Input: part model. Units: mm. Frame: model coordinates. Face numbers are marked on the shaded views. A direction names the side the tool comes from. Coordinates: 2 decimals unless noted, no trailing zeros. Loops run counter-clockwise (first coordinate to the right, second up) from the corner with the lowest first, then second, coordinate; pieces in that order, holes last.
Item 1: Reachability of the marked faces 3 and 4 from +Z, -Z, +X, -X, +Y, -Y: full face, straight path, thin tool, end or side. Return the list, or none.
Item 2: Section A-A on y = 32. Return loops of the section in (x, z).
Item 3: Pull-direction query (Z, two-part tool) for the marked faces 1 and 2; classes: released by +Z, released by -Z, zero draft, split by the parting line, or undercut.
Item 4: Ray query, line 1 along X through (y, z) = (94.5, 0); line 2 along X through (y, z) = (29, 0); line 3 along Z through (x, y) = (-4.5, 85.5). Return the intervals inside material, ascending.
Item 5: Contact query for flat-ended pins moving along their axis: P1, Ø22, axis at x = 0, z = 0, coming from the -Y side; P2, Ø5, axis at x = 18.5, z = -14, coming from the +Y side; P3, Ø5, axis at x = 19.5, z = 7, coming from the -Y side; P4, Ø10, axis at y = 82.5, z = 3, coming from the +X side. Output: stop coordinate, or through.
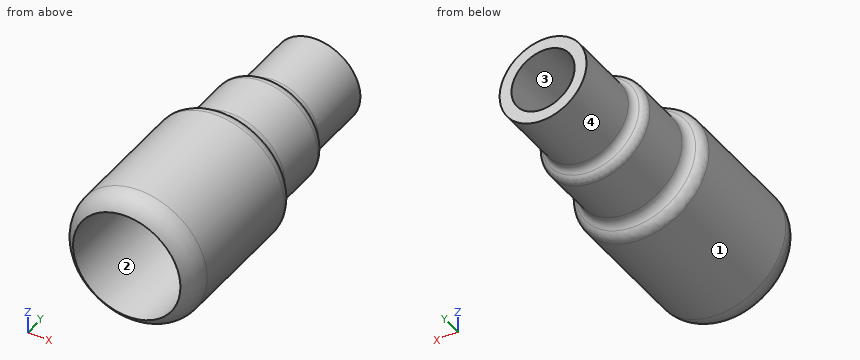
```python
from build123d import *

# Parameters (mm, degrees)
SKETCH_1_R      = 26
SKETCH_1_R_2    = 21
EXTRUDE_1_DEPTH = 60
FILLET_1_R      = 10
EXTRUDE_START   = -2
SKETCH_2_R      = 21
SKETCH_2_R_2    = 12.35
EXTRUDE_2_DEPTH = 30
SKETCH_3_R      = 17
SKETCH_3_R_2    = 12.35
EXTRUDE_3_DEPTH = 30
FILLET_3_R      = 4
FILLET_4_R      = 4
FILLET_6_R      = 5
FILLET_7_R      = 5
FILLET_8_R      = 5
FILLET_9_R      = 5


# Some blends are built 0.0001 mm under size
with BuildPart() as part:
    # Эскиз1 → Вытянуть1 (new body)
    with BuildSketch(Plane(origin=(0, 0, 0), x_dir=(1, 0, 0), z_dir=(0, 1, 0))):
        with Locations(Location((0, 0, 0), (0, 0, 270))):
            Circle(SKETCH_1_R)
        with Locations(Location((0, 0, 0), (0, 0, 270))):
            Circle(SKETCH_1_R_2, mode=Mode.SUBTRACT)
    extrude(amount=EXTRUDE_1_DEPTH)

    # Скругление1
    # the kernel refuses this fillet: 10 mm, written as the material it takes off along each edge
    with BuildSketch(Plane(origin=(0, 0, 0), x_dir=(0, 0, 1), z_dir=(-1, 0, 0))) as fillet_1_piece_1:
        with BuildLine():
            CenterArc((16, 8.660254038), FILLET_1_R, 300, 60)
            Line((21, 0), (21.1, -0.173205081))
            ThreePointArc((21.1, -0.173205081), (23.5, -0.2), (26, -0.2))
            Line((26, -0.2), (26.2, 0))
            Line((26.2, 0), (26.2, 8.660254038))
            Line((26.2, 8.660254038), (26, 8.660254038))
        make_face()
    revolve(axis=Axis((0, 0, 0), (0, 1, 0)), mode=Mode.SUBTRACT)

    # Эскиз2 → Вытянуть2 (add)
    with BuildSketch(Plane(origin=(0, 60, 0), x_dir=(1, 0, 0), z_dir=(0, 1, 0)).offset(EXTRUDE_START)):
        with Locations(Location((0, 0, 0), (0, 0, 270))):
            Circle(SKETCH_2_R)
        with Locations(Location((0, 0, 0), (0, 0, 270))):
            Circle(SKETCH_2_R_2, mode=Mode.SUBTRACT)
    extrude(amount=EXTRUDE_2_DEPTH)

    # Эскиз3 → Вытянуть3 (add)
    with BuildSketch(Plane(origin=(0, 88, 0), x_dir=(1, 0, 0), z_dir=(0, 1, 0))):
        with Locations(Location((0, 0, 0), (0, 0, 270))):
            Circle(SKETCH_3_R)
        with Locations(Location((0, 0, 0), (0, 0, 270))):
            Circle(SKETCH_3_R_2, mode=Mode.SUBTRACT)
    extrude(amount=EXTRUDE_3_DEPTH)

    # Скругление3
    fillet_3_edges = [part.edges().sort_by_distance(p)[0] for p in [
        (0, 88, -17),
    ]]
    fillet(fillet_3_edges, radius=FILLET_3_R - 0.0001)  # a hair under: the kernel refuses the full size

    # Скругление4
    fillet_4_edges = [part.edges().sort_by_distance(p)[0] for p in [
        (0, 88, -21),
    ]]
    fillet(fillet_4_edges, radius=FILLET_4_R)

    # Скругление6
    fillet_6_edges = [part.edges().sort_by_distance(p)[0] for p in [
        (0, 60, -21),
    ]]
    fillet(fillet_6_edges, radius=FILLET_6_R - 0.0001)  # a hair under: the kernel refuses the full size

    # Скругление7
    fillet_7_edges = [part.edges().sort_by_distance(p)[0] for p in [
        (0, 60, -26),
    ]]
    fillet(fillet_7_edges, radius=FILLET_7_R)

    # Скругление8
    fillet_8_edges = [part.edges().sort_by_distance(p)[0] for p in [
        (0, 58, -21),
    ]]
    fillet(fillet_8_edges, radius=FILLET_8_R)

    # Скругление9
    fillet_9_edges = [part.edges().sort_by_distance(p)[0] for p in [
        (0, 58, -12.35),
    ]]
    fillet(fillet_9_edges, radius=FILLET_9_R)


solid = part.part
```
Results found:
1. face 3: +Y, -Y
1. face 4: +Y
2. outline: circle Ø52 at (0, 0); hole circle Ø42 at (0, 0)
3. face 1: split by the parting line
3. face 2: undercut
4. line 1: x = -17 to -12.35, 12.35 to 17
4. line 2: x = -26 to -21, 21 to 26
4. line 3: z = -20.49 to -11.5, 11.5 to 20.49
5. P1: passes through
5. P2: stops at y = 86.59
5. P3: stops at y = 0
5. P4: stops at x = 21
